Model file for the job. Use its own axes, mm. Face numbers are marked on the shaded views. A direction names the side the tool comes from. Give positions to 0.01 mm unless a question says otherwise; leave off trailing zeros. Loops run counter-clockwise (first coordinate to the right, second up) from the corner with the lowest first, then second, coordinate; pieces in that order, holes last. Notation, with made-up numbers: M 51,47.25 L 89,47.25 A9 ccw 89,56.25 Z; hole C 60,65 d4. An arc over 180 degrees is marked long. Answer in a Markdown table with one row per item.
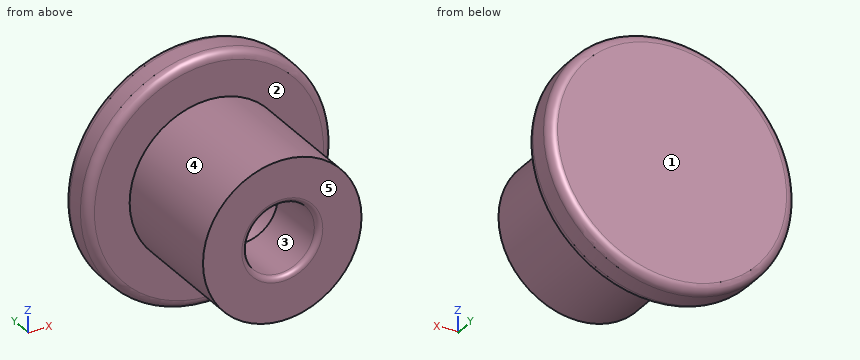
```python
from build123d import *

# Parameters (mm, degrees)
SKETCH1_R                              = 3.5
BOSS_EXTRUDE1_DEPTH                    = 1
SKETCH3_R                              = 2.25
BOSS_EXTRUDE3_DEPTH                    = 3.5
FILLET1_R                              = 0.25
F_1_16_0_07874016_DIAMETER_HOLE1_D     = 2.000000064
F_1_16_0_07874016_DIAMETER_HOLE1_DEPTH = 1.899139362
F_1_16_0_07874016_DIAMETER_HOLE1_TIP   = 0.600860638
FILLET2_R                              = 0.15


with BuildPart() as part:
    # Sketch1 → Boss-Extrude1 (new body)
    with BuildSketch(Plane(origin=(0, 0, 0), x_dir=(1, 0, 0), z_dir=(0, 1, 0))):
        with Locations(Location((0, 0, 0), (0, 0, 270))):
            Circle(SKETCH1_R)
    extrude(amount=BOSS_EXTRUDE1_DEPTH)

    # Sketch3 → Boss-Extrude3 (add)
    with BuildSketch(Plane.XZ):
        with Locations(Location((0, 0, 0), (0, 0, 270))):
            Circle(SKETCH3_R)
    extrude(amount=BOSS_EXTRUDE3_DEPTH)

    # Fillet1
    fillet1_edges = [part.edges().sort_by_distance(p)[0] for p in [
        (0, 0, -3.5),
        (0, 1, -3.5),
    ]]
    fillet(fillet1_edges, radius=FILLET1_R)

    # 1/16 (0.07874016) Diameter Hole1
    with Locations(Plane(origin=(0, -3.5, 0), x_dir=(-1, 0, 0), z_dir=(0, -1, 0))):
        with Locations((0, 0)):
            Hole(F_1_16_0_07874016_DIAMETER_HOLE1_D / 2, depth=F_1_16_0_07874016_DIAMETER_HOLE1_DEPTH)
            with Locations((0, 0, -(F_1_16_0_07874016_DIAMETER_HOLE1_DEPTH + F_1_16_0_07874016_DIAMETER_HOLE1_TIP / 2))):  # 118° drill point
                Cone(0, F_1_16_0_07874016_DIAMETER_HOLE1_D / 2, F_1_16_0_07874016_DIAMETER_HOLE1_TIP, mode=Mode.SUBTRACT)

    # Fillet2
    fillet2_edges = [part.edges().sort_by_distance(p)[0] for p in [
        (-1.000000032, -3.5, 0),
    ]]
    fillet(fillet2_edges, radius=FILLET2_R)


solid = part.part
```
Q1. Probe probe 1 along X at (y, z) = (-2.75, 0); probe 2 along Y at (x, z) = (0.5, -2.5); probe 3 along Z at (x, y) = (-0.25, -2.75). List the from-to ranges inside material, lowest first.
Reported:
| item | result |
|---|---|
| probe 1 | -2.25 to -1, 1 to 2.25 |
| probe 2 | 0 to 1 |
| probe 3 | -2.24 to -0.97, 0.97 to 2.24 |
Q2. Drop flat-ended pins along their axis: pin 1 (1 mm diameter, centred on y = -2.5, z = 1, fed in from -X); pin 2 (2 mm diameter, centred on x = 1, y = -2, fed in from -Z). Give the stop position or say it passes through.
Reported:
| item | result |
|---|---|
| pin 1 | x = -2.19 |
| pin 2 | z = -2.25 |
Q3. Saw through at A-A (y = -2.8). Give the cut face in (x, z).
Reported:
| item | result |
|---|---|
| outline | C 0,0 d4.5; hole C 0,0 d2 |
Q4. Saw through at B-B (y = -0.9). Give the cut face in (x, z), and give its area (3 significant figures).
Reported:
| item | result |
|---|---|
| outline | C 0,0 d4.5 |
| area | 15.9 mm² |
Q5. 3-axis set-ups, long thin cutter, end or side, ignore diameter. For the marked faces 1 and 2: which of +Z, -Z, +X, -X, +Y, -Y reach the whole face in a straight line?
Reported:
| item | result |
|---|---|
| face 1 | +Z, -Z, +X, -X, +Y |
| face 2 | -Y |
Q6. Mould opens along X. For the marked faces 3, 4 and 5 say: released by +X, released by -X, zero draft, split by the parting line, or undercut.
Reported:
| item | result |
|---|---|
| face 3 | undercut |
| face 4 | split by the parting line |
| face 5 | zero draft |
